Check sheet for the modelled part. Datum: model origin and axes. Units: mm. A direction names the side the tool comes from. Coordinates: 2 decimals unless noted, no trailing zeros. Loops run counter-clockwise (first coordinate to the right, second up) from the corner with the lowest first, then second, coordinate; pieces in that order, holes last. Notation, with made-up numbers: (83, -0.5) - (141, -0.5) arc R36 cw to (141, 35.5) - close; hole circle Ø6 at (-29.5, -4). An arc over 180 degrees is marked (long way). Use a Markdown table: item, result. Add a question column.
1) Draft check along Y on faces 1 (the cylindrical face through (83.661, 28.673, 3.193)), 2 (the flat face through (-86, 21.844, 3)), 3 (the flat face through (-1, 1, 6.477)), 4 (the flat face through (-86, -18.796, 3)). Enter one of: pulls with the +Y half, pulls with the -Y half, needs draft (parallel to the pull), parting line crosses it, or undercut.
2) Tool access check on faces 5 (the flat face through (-88.773, -12, 3)), 6 (the flat face through (-88.773, 32, 3)), 7 (the flat face through (-95.25, 0, 3)), 8 (the flat face through (-86, -21.844, 3)). Record the directions out of +Z, -Z, +X, -X, +Y, -Y that give a thin tool (end or side, any length) a straight path to the whole face; none if there is none.
3) Sectioned sample at B-B, the plane y = 35. Enter the section's corners in (x, z).
4) Go/stop test with flat-tipped pins: P1, Ø3, axis at x = -93.5, z = 2.5, coming from the -Y side; P2, Ø3, axis at y = 34, z = 4.5, coming from the -X side; P3, Ø1, axis at y = 21, z = 2.5, coming from the -X side. Record where each tip stops, or that it passes through.
5) Sectioned sample at A-A, the plane y = 2.5. Enter the section's corners in (x, z).
6) Sectioned sample at C-C, the plane y = -26.5. Enter the section's corners in (x, z).
7) Thickness scan on line 1 (Y direction, x = -85.5, z = 5.75); line 2 (Y direction, x = 54.61, z = 5.25); line 3 (Y direction, x = 59, z = 1.5). Record the ranges inside material, lowest first.
from build123d import *

# Parameters (mm, degrees)
SKETCH1_R           = 6.35
BOSS_EXTRUDE1_DEPTH = 6.477


with BuildPart() as part:
    # Sketch1 → Boss-Extrude1 (new body)
    with BuildSketch(Plane.XY):
        with BuildLine():
            Line((-88.773, 18.796), (-88.773, 6.35))
            Line((-88.773, 6.35), (-95.25, 6.35))
            Line((-95.25, 6.35), (-95.25, -6.35))
            Line((-95.25, -6.35), (-88.773, -6.35))
            Line((-88.773, -6.35), (-88.773, -18.796))
            Line((-88.773, -18.796), (-82.423, -18.796))
            Line((-82.423, -18.796), (-82.423, -17.145))
            Line((-82.423, -17.145), (-79.883, -17.145))
            Line((-79.883, -17.145), (-79.883, -18.796))
            Line((-79.883, -18.796), (-69.723, -18.796))
            Line((-69.723, -18.796), (-69.723, -21.844))
            Line((-69.723, -21.844), (-79.883, -21.844))
            Line((-79.883, -21.844), (-79.883, -23.495))
            Line((-79.883, -23.495), (-82.423, -23.495))
            Line((-82.423, -23.495), (-82.423, -21.844))
            Line((-82.423, -21.844), (-88.773, -21.844))
            Line((-88.773, -21.844), (-88.773, -40.894))
            Line((-88.773, -40.894), (54.61, -40.894))
            ThreePointArc((54.61, -40.894), (83.346819587, -28.990819587), (95.25, -0.254))
            Line((95.25, -0.254), (95.25, 0.254))
            ThreePointArc((95.25, 0.254), (83.346819587, 28.990819587), (54.61, 40.894))
            Line((54.61, 40.894), (-88.773, 40.894))
            Line((-88.773, 40.894), (-88.773, 21.844))
            Line((-88.773, 21.844), (-82.423, 21.844))
            Line((-82.423, 21.844), (-82.423, 23.495))
            Line((-82.423, 23.495), (-79.883, 23.495))
            Line((-79.883, 23.495), (-79.883, 21.844))
            Line((-79.883, 21.844), (-69.723, 21.844))
            Line((-69.723, 21.844), (-69.723, 18.796))
            Line((-69.723, 18.796), (-79.883, 18.796))
            Line((-79.883, 18.796), (-79.883, 17.145))
            Line((-79.883, 17.145), (-82.423, 17.145))
            Line((-82.423, 17.145), (-82.423, 18.796))
            Line((-82.423, 18.796), (-88.773, 18.796))
        make_face()
        with Locations((54.61, 0)):
            Circle(SKETCH1_R, mode=Mode.SUBTRACT)
    extrude(amount=BOSS_EXTRUDE1_DEPTH)


solid = part.part
Solved:
| question | item | result |
|---|---|---|
| 1 | face 1 | pulls with the +Y half |
| 1 | face 2 | undercut |
| 1 | face 3 | needs draft |
| 1 | face 4 | undercut |
| 2 | face 5 | +Z, -Z, -X, -Y |
| 2 | face 6 | +Z, -Z, -X, +Y |
| 2 | face 7 | +Z, -Z, -X, +Y, -Y |
| 2 | face 8 | +Z, -Z, -X |
| 3 | outline | (-88.77, 0) - (75.69, 0) - (75.69, 6.48) - (-88.77, 6.48) - close |
| 4 | P1 | stops at y = -6.35 |
| 4 | P2 | stops at x = -88.77 |
| 4 | P3 | stops at x = -69.72 |
| 5 | outline | (-95.25, 0) - (48.77, 0) - (48.77, 6.48) - (-95.25, 6.48) - close; (60.45, 0) - (95.19, 0) - (95.19, 6.48) - (60.45, 6.48) - close |
| 6 | outline | (-88.77, 0) - (85.64, 0) - (85.64, 6.48) - (-88.77, 6.48) - close |
| 7 | line 1 | y = -40.89 to -21.84, -18.8 to 18.8, 21.84 to 40.89 |
| 7 | line 2 | y = -40.89 to -6.35, 6.35 to 40.89 |
| 7 | line 3 | y = -40.66 to -4.59, 4.59 to 40.66 |
